Autodesk Inventor part; units mm, degrees
ref_plane "YZ Plane" through (0, 0, 0) normal (1, 0, 0) x (0, 1, 0)
ref_plane "XZ Plane" through (0, 0, 0) normal (0, 1, 0) x (-1, 0, 0)
ref_plane "XY Plane" through (0, 0, 0) normal (0, 0, 1) x (1, 0, 0)
sketch "Sketch1" plane through (0, 0, 0) normal (0, 0, 1) x (1, 0, 0)
  line L0 (0, 0) -> (228.6, 0)
  line L1 (228.6, 0) -> (228.6, -203.2)
  line L2 (228.6, -203.2) -> (0, -203.2)
  line L3 (0, -203.2) -> (0, 0)
  dimension "d0" = 228.6
  dimension "d1" = 203.2
extrude "Extrusion1" add sketch "Sketch1" along normal blind 3.175
sketch "Sketch2" plane through (0, 0, 3.175) normal (0, 0, 1) x (1, 0, 0)
  circle A0 centre (78.105, -184.15) radius 3.3734
  circle A1 centre (150.495, -184.15) radius 3.3734
  line L0 (0, -203.2) -> (228.6, -203.2)
  line L1 (0, 0) -> (0, -203.2)
  dimension "d4" = 6.7469
  dimension "d5" = 6.7469
  dimension "d6" = 19.05
  dimension "d7" = 19.05
  dimension "d8" = 72.39
  dimension "d9" = 78.105
extrude "Extrusion2" cut sketch "Sketch2" against normal blind 3.175
properties part number "plate"
Input: part model. Units: mm. Frame: model coordinates. Give positions to 0.01 mm unless a question says otherwise; leave off trailing zeros. Order: outer loops, then holes, each group sorted by start corner. A loop starts at its lowest first (then second) coordinate and runs counter-clockwise, first axis right, second up. Notation, with made-up numbers: M 22,-2 L 28,-2 A10 ccw 28,10 Z; hole C 10,1 d3. An arc over 180 degrees is marked long. One line per question, with ' | ' between items. Start each with the question number.
1. First-contact query: pin 1 Ø6 at (x, y) = (78.105, -184.15) entering from +Z. Flat tip, straight axial feed; report the tip coordinate or a pass-through.
2. Section query A-A (y = -184.15). Return the cut outline in (x, z) (3 decimals).
3. Pull-direction query (X, two-part tool) for faces 1 (the face through (79.662, -187.143, 1.61)), 2 (the face through (113, -100, 3.175)); classes: released by +X, released by -X, zero draft, split by the parting line, or undercut.
4. Material intervals for probe 1 along X at (y, z) = (-184.15, 1.05); probe 2 along X at (y, z) = (-187, 0.95), sorted ascending. Write a range as [from, to].
Here are the results:
1) pin 1: through
2) outline: M 0,0 L 74.732,0 L 74.732,3.175 L 0,3.175 Z; M 81.478,0 L 147.122,0 L 147.122,3.175 L 81.478,3.175 Z; M 153.868,0 L 228.6,0 L 228.6,3.175 L 153.868,3.175 Z
3) face 1: undercut | face 2: zero draft
4) probe 1: [0, 74.73], [81.48, 147.12], [153.87, 228.6] | probe 2: [0, 76.3], [79.91, 148.69], [152.3, 228.6]
